```python
from build123d import *
from build123d.topology import SkipClean

# Parameters (mm, degrees)
SKETCH1_R           = 17.4625
BOSS_EXTRUDE1_DEPTH = 5.08
CUT_EXTRUDE1_DEPTH  = 5.08
SKETCH3_R           = 3.175
BOSS_EXTRUDE2_DEPTH = 0.254
SKETCH4_R           = 0.8255
CUT_EXTRUDE2_DEPTH  = 6.334
SKETCH5_R           = 12.7
SKETCH5_R_2         = 6.35
CUT_EXTRUDE3_DEPTH  = 2.54
SKETCH6_R           = 12.7
SKETCH6_R_2         = 6.35
CUT_EXTRUDE4_DEPTH  = 0.635
SKETCH7_R           = 6.35
SKETCH7_R_2         = 3.175
CUT_EXTRUDE5_DEPTH  = 1.905


with BuildPart() as part:
    # Sketch1 → Boss-Extrude1 (new body)
    with BuildSketch(Plane.XY):
        Circle(SKETCH1_R)
    extrude(amount=BOSS_EXTRUDE1_DEPTH)

    # Sketch2 → Cut-Extrude1 (cut)
    with BuildSketch(Plane(origin=(0, 0, 0), x_dir=(-1, 0, 0), z_dir=(0, 0, -1))):
        with BuildLine():
            Line((2.205331856, -12.507058463), (1.102665928, -6.253529232))
            ThreePointArc((1.102665928, -6.253529232), (3.732436352, -5.137257914), (5.606717215, -2.981144424))
            Line((5.606717215, -2.981144424), (11.213434429, -5.962288847))
            ThreePointArc((11.213434429, -5.962288847), (7.464872704, -10.274515829), (2.205331856, -12.507058463))
        make_face()
        with BuildLine():
            Line((-1.102665928, -6.253529232), (-2.205331856, -12.507058463))
            ThreePointArc((-2.205331856, -12.507058463), (-7.464872704, -10.274515829), (-11.213434429, -5.962288847))
            Line((-11.213434429, -5.962288847), (-5.606717215, -2.981144424))
            ThreePointArc((-5.606717215, -2.981144424), (-3.732436352, -5.137257914), (-1.102665928, -6.253529232))
        make_face()
        with BuildLine():
            Line((-6.288202237, -0.883749191), (-12.576404473, -1.767498382))
            ThreePointArc((-12.576404473, -1.767498382), (-12.078417757, 3.924515829), (-9.135615464, 8.822161305))
            Line((-9.135615464, 8.822161305), (-4.567807732, 4.411080652))
            ThreePointArc((-4.567807732, 4.411080652), (-6.039208878, 1.962257914), (-6.288202237, -0.883749191))
        make_face()
        with BuildLine():
            Line((-2.783656782, 5.707342194), (-5.567313564, 11.414684388))
            ThreePointArc((-5.567313564, 11.414684388), (0, 12.7), (5.567313564, 11.414684388))
            Line((5.567313564, 11.414684388), (2.783656782, 5.707342194))
            ThreePointArc((2.783656782, 5.707342194), (0, 6.35), (-2.783656782, 5.707342194))
        make_face()
        with BuildLine():
            Line((4.567807732, 4.411080652), (9.135615464, 8.822161305))
            ThreePointArc((9.135615464, 8.822161305), (12.078417757, 3.924515829), (12.576404473, -1.767498382))
            Line((12.576404473, -1.767498382), (6.288202237, -0.883749191))
            ThreePointArc((6.288202237, -0.883749191), (6.039208878, 1.962257914), (4.567807732, 4.411080652))
        make_face()
    extrude(amount=-CUT_EXTRUDE1_DEPTH, mode=Mode.SUBTRACT)

    # Sketch3 → Boss-Extrude2 (add)
    with BuildSketch(Plane.XY.offset(5.08)):
        Circle(SKETCH3_R)
    extrude(amount=BOSS_EXTRUDE2_DEPTH)

    # Sketch4 → Cut-Extrude2 (cut, through all)
    with BuildSketch(Plane.XY.offset(5.334)):
        Circle(SKETCH4_R)
    extrude(amount=-CUT_EXTRUDE2_DEPTH, mode=Mode.SUBTRACT)

    # Sketch5 → Cut-Extrude3 (cut)
    with BuildSketch(Plane.XY.offset(5.08)):
        with Locations(Location((0, 0, 0), (0, 0, 180))):  # turned: the seam where the file's is
            Circle(SKETCH5_R)
        with Locations(Location((0, 0, 0), (0, 0, 180))):  # turned: the seam where the file's is
            Circle(SKETCH5_R_2, mode=Mode.SUBTRACT)
    extrude(amount=-CUT_EXTRUDE3_DEPTH, mode=Mode.SUBTRACT)

    # Sketch6 → Cut-Extrude4 (cut)
    with SkipClean():  # keep this step's faces unmerged: merging them makes the solid invalid here
        with BuildSketch(Plane(origin=(0, 0, 0), x_dir=(-1, 0, 0), z_dir=(0, 0, -1))):
            Circle(SKETCH6_R)
            Circle(SKETCH6_R_2, mode=Mode.SUBTRACT)
        extrude(amount=-CUT_EXTRUDE4_DEPTH, mode=Mode.SUBTRACT)

    # Sketch7 → Cut-Extrude5 (cut)
    with SkipClean():  # keep this step's faces unmerged: merging them makes the solid invalid here
        with BuildSketch(Plane.XY.offset(5.08)):
            with Locations(Location((0, 0, 0), (0, 0, 180))):  # turned: the seam where the file's is
                Circle(SKETCH7_R)
            Circle(SKETCH7_R_2, mode=Mode.SUBTRACT)
        extrude(amount=-CUT_EXTRUDE5_DEPTH, mode=Mode.SUBTRACT)


solid = part.part
```
The model under review builds one solid part; all positions refer to its coordinate system, in mm. A direction names the side the tool comes from. Round coordinates to 2 decimals unless told otherwise and drop trailing zeros. Order: outer loops, then holes, each group sorted by start corner. A loop starts at its lowest first (then second) coordinate and runs counter-clockwise, first axis right, second up. Notation, with made-up numbers: (70, 8.5) -> (87, 8.5) arc R20 cw to (87, 37.5) -> close; hole circle Ø11 at (46, -20.75). An arc over 180 degrees is marked (long way). One line per item, written item: value. Start each with the question number.
Q1. Take a section at A-A (y = 0). Count the separate pieces of the cut face and the enclosed holes in it, and give its area (3 significant figures).
Q2. Clearance check with flat-ended pins moving along their axes: pin 1 Ø12 at (x, y) = (12, -12.5) entering from +Z; pin 2 Ø5 at (x, y) = (2, -8) entering from +Z (3 decimals); pin 3 Ø2.5 at (x, y) = (8.5, -4.5) entering from -Z (3 decimals); pin 4 Ø2 at (x, y) = (-5, -8.5) entering from -Z. State where each tip first meets the part, or that it passes through.
Q3. Wall thickness on line 1 (Y direction, x = 0, z = 3.05); line 2 (Y direction, x = 0, z = 1.7); line 3 (X direction, y = 8.5, z = 2.35): over which ranges is each line inside the solid? List them lowest first.
Q4. Take a section at D-D (x = -5). Write out the cut boundary in (y, z) (3 decimals).
Q5. Mouldability with a two-part tool opening along X and no side actions: class faces 1 (the face through (1, -13, 0)), 2 (the face through (-13.858, -10.626, 2.504)), 3 (the face through (6, 8, 0.635)) as released by +X, released by -X, zero draft, split by the parting line, or undercut.
Q6. Machinability: for faces 4 (the face through (9.39, -1.32, 1.57)), 5 (the face through (-9, -3, 2.54)), 6 (the face through (0, -1, 0)), 7 (the face through (1, -1, 5.334)), 8 (the face through (9, -3, 0.635)), which of the approach directions +Z, -Z, +X, -X, +Y, -Y give a long, thin tool a straight path to every point of the face, cutting with its end or side? Answer none if there is none.
Reported:
1. separate pieces: 4
1. enclosed holes: 0
1. area: 93.6 mm2
2. pin 1: stops at z = 5.08
2. pin 2: stops at z = 3.175
2. pin 3: stops at z = 0.635
2. pin 4: passes through
3. line 1: y = -17.46 to -12.7, -6.35 to -0.83, 0.83 to 6.35, 12.7 to 17.46
3. line 2: y = -17.46 to -0.83, 0.83 to 6.35, 12.7 to 17.46
3. line 3: x = -15.25 to -9.44, -8.8 to -4.15, 4.15 to 8.8, 9.44 to 15.25
4. outline: (-16.731, 0) -> (-11.674, 0) -> (-11.674, 5.08) -> (-16.731, 5.08) -> close; (-3.914, 0) -> (3.914, 0) -> (3.914, 3.175) -> (-3.914, 3.175) -> close; (4.828, 0.635) -> (10.252, 0.635) -> (10.252, 2.54) -> (4.828, 2.54) -> close; (11.674, 0) -> (16.731, 0) -> (16.731, 5.08) -> (11.674, 5.08) -> close
5. face 1: zero draft
5. face 2: split by the parting line
5. face 3: undercut
6. face 4: +Z, -Z
6. face 5: +Z
6. face 6: -Z, +X, -X, +Y, -Y
6. face 7: +Z, +X, -X, +Y, -Y
6. face 8: -Z
